from build123d import *

# Parameters (mm, degrees)
SKETCH1_R           = 1.905
BOSS_EXTRUDE3_DEPTH = 6.35
FILLET4_R           = 3.81


with BuildPart() as part:
    # Sketch1 → Boss-Extrude3 (new body)
    with BuildSketch(Plane(origin=(0, 0, 0), x_dir=(1, 0, 0), z_dir=(0, 1, 0))):
        Polygon((-65.88775931, 11.594773286), (-65.88775931, -13.805226714), (-23.03795931, -13.805226714), (-21.76795931, -11.265226714), (-20.49795931, -13.805226714), (-3.97525931, -13.805226714), (-3.97525931, 11.594773286), (-20.49795931, 11.594773286), (-21.76795931, 9.054773286), (-23.03795931, 11.594773286), align=None)
        with Locations(Location((-57.421862263, -5.339329667, 0), (0, 0, 270))):
            Circle(SKETCH1_R, mode=Mode.SUBTRACT)
        with Locations(Location((-48.953147413, 3.129385183, 0), (0, 0, 270))):
            Circle(SKETCH1_R, mode=Mode.SUBTRACT)
    extrude(amount=BOSS_EXTRUDE3_DEPTH)

    # Fillet4
    fillet4_edges = [part.edges().sort_by_distance(p)[0] for p in [
        (-23.03795931, 3.175, -11.594773286),
        (-20.49795931, 3.175, -11.594773286),
        (-3.97525931, 3.175, -11.594773286),
        (-3.97525931, 3.175, 13.805226714),
        (-20.49795931, 3.175, 13.805226714),
        (-23.03795931, 3.175, 13.805226714),
        (-65.88775931, 3.175, 13.805226714),
        (-65.88775931, 3.175, -11.594773286),
    ]]
    fillet(fillet4_edges, radius=FILLET4_R)


solid = part.part
Verification items for the finished model (mm, model axes). A direction names the side the tool comes from. Coordinates: 2 decimals unless noted, no trailing zeros. Loops run counter-clockwise (first coordinate to the right, second up) from the corner with the lowest first, then second, coordinate; pieces in that order, holes last. Notation, with made-up numbers: (89.25, -25.75) -> (106.25, -25.75) arc R25 cw to (106.25, -0.75) -> close; hole circle Ø1 at (48, -40). An arc over 180 degrees is marked (long way). Write each question's results on one line, items separated by ' | '.
Item 1: Section check D-D, the plane x = -20. Enter the section's corners in (y, z), plus the area to 3 significant figures.
Found:
outline: (0, -11.11) -> (6.35, -11.11) -> (6.35, 13.32) -> (0, 13.32) -> close | area: 155 mm2
Item 2: Tool access check on faces 1 (the face through (-20.17, 3.22, -11.01)), 2 (the face through (-5.1, 3.2, 12.7)), 3 (the face through (-23.41, 3.22, 13.25)). Record the directions out of +Z, -Z, +X, -X, +Y, -Y that give a thin tool (end or side, any length) a straight path to the whole face; none if there is none.
Found:
face 1: -Z, +Y, -Y | face 2: +Z, +X, +Y, -Y | face 3: +Z, +Y, -Y
Item 3: Section check A-A, the plane z = -3.25. Enter the section's corners in (x, y).
Found:
outline: (-65.89, 0) -> (-50.85, 0) -> (-50.85, 6.35) -> (-65.89, 6.35) -> close; (-47.05, 0) -> (-3.98, 0) -> (-3.98, 6.35) -> (-47.05, 6.35) -> close
Item 4: Mould release check, pull along X, two halves, no side actions. Record for faces 4 (the face through (-3.975, 3, 1)), 5 (the face through (-13, 3, -11.595)), 6 (the face through (-59.282, 3.131, 4.926)): +X half, -X half, draft (parallel to the pull), parting line (faces both ways), or undercut.
Found:
face 4: +X half | face 5: draft | face 6: undercut
Item 5: Material ranges on L1, parallel to X at y = 4.5, z = -9.5; L2, parallel to X at y = 1.25, z = 10.25; L3, parallel to X at y = 3.5, z = -1.5, recorded low to high.
Found:
L1: x = -65.48 to -21.99, -21.55 to -4.38 | L2: x = -65.88 to -3.98 | L3: x = -65.89 to -49.94, -47.97 to -3.98
Item 6: Section check B-B, the plane x = -58.5. Enter the section's corners in (y, z).
Found:
outline: (0, -11.59) -> (6.35, -11.59) -> (6.35, 3.77) -> (0, 3.77) -> close; (0, 6.91) -> (6.35, 6.91) -> (6.35, 13.81) -> (0, 13.81) -> close
Item 7: Section check C-C, the plane y = 5.5. Enter the section's corners in (x, z) (3 decimals).
Found:
outline: (-65.888, -7.785) arc R3.81 ccw to (-62.078, -11.595) -> (-25.393, -11.595) arc R3.81 ccw to (-21.985, -9.489) -> (-21.768, -9.055) -> (-21.551, -9.489) arc R3.81 ccw to (-18.143, -11.595) -> (-7.785, -11.595) arc R3.81 ccw to (-3.975, -7.785) -> (-3.975, 9.995) arc R3.81 ccw to (-7.785, 13.805) -> (-18.143, 13.805) arc R3.81 ccw to (-21.551, 11.699) -> (-21.768, 11.265) -> (-21.985, 11.699) arc R3.81 ccw to (-25.393, 13.805) -> (-62.078, 13.805) arc R3.81 ccw to (-65.888, 9.995) -> close; hole circle Ø3.81 at (-57.422, 5.339); hole circle Ø3.81 at (-48.953, -3.129)
Item 8: Gauge pin test, flat end, axial feed: pin 1 (1 mm diameter, centred on y = 3, z = 11, fed in from -X). Record the tip position at first contact, or that the pin passes through.
Found:
pin 1: stops at x = -65.85
